Design review of the part built by this model. Coordinates are the model's own, in mm. Face numbers are marked on the shaded views. A direction names the side the tool comes from. Round coordinates to 2 decimals unless told otherwise and drop trailing zeros. Write each loop counter-clockwise with the first axis right and the second up, starting at its lowest first coordinate (ties: lowest second). Pieces come first, ordered by that corner, then holes. Notation, with made-up numbers: M 82.5,66 L 100.5,66 A29 ccw 100.5,98 Z; hole C -35.75,-25 d7. An arc over 180 degrees is marked long. One line per question, with ' | ' between items. Start each with the question number.
Item 1: Machinability: for the marked faces 4 and 5, which of the approach directions +Z, -Z, +X, -X, +Y, -Y give a long, thin tool a straight path to every point of the face, cutting with its end or side? Answer none if there is none.
Item 2: Add section D-D, the plane x = 27.5. State the section outline as (y, z) points, and give its area (3 significant figures).
Item 3: For L1, parallel to X at y = 6.25, z = -17; L2, parallel to Z at x = -14, y = 19.5; L3, parallel to Z at x = -19.5, y = 15.75, list the stretches that pass through material, from the lowest coordinate up.
Item 4: Add section A-A, the plane z = 0. State the section outline as (x, y) points, and give its area (3 significant figures).
Item 5: Draft analysis for pull direction Z (two halves, no side actions). For the marked faces 1, 2 and 3, state which applies: released by +Z, released by -Z, zero draft, split by the parting line, or undercut.
Item 6: Insertion check: pin 1 Ø2.5 at (y, z) = (9.5, -24.5) entering from +X; pin 2 Ø5 at (y, z) = (13, 24.5) entering from +X; pin 3 Ø1.4 at (y, z) = (18, 24) entering from -X. Each pin has a flat end and moves straight along its axis. Give the tip position at first contact, or say it passes through.
Item 7: Add section B-B, the plane y = 7.25. Give the number of separate pieces and of enclosed holes in the cut face, and give its area (3 significant figures).
Item 8: Add section C-C, the plane x = 4.5. State the section outline as (y, z) points, and give its area (3 significant figures).
```python
from build123d import *

# Parameters (mm, degrees)
SKETCH1_R           = 2.01295
BOSS_EXTRUDE1_DEPTH = 25.4


with BuildPart() as part:
    # Sketch1 → Boss-Extrude1 (new body)
    with BuildSketch(Plane(origin=(0, 0, 0), x_dir=(1, 0, 0), z_dir=(0, 1, 0))):
        with BuildLine():
            ThreePointArc((32.16275, -21.451406337), (28.205815008, -27.54883493), (22.589075945, -32.16275))
            Line((22.589075945, -32.16275), (-22.589075945, -32.16275))
            ThreePointArc((-22.589075945, -32.16275), (-28.205815008, -27.54883493), (-32.16275, -21.451406337))
            Line((-32.16275, -21.451406337), (-32.16275, 21.451406337))
            ThreePointArc((-32.16275, 21.451406337), (-28.205815008, 27.54883493), (-22.589075945, 32.16275))
            Line((-22.589075945, 32.16275), (22.589075945, 32.16275))
            ThreePointArc((22.589075945, 32.16275), (28.205815008, 27.54883493), (32.16275, 21.451406337))
            Line((32.16275, 21.451406337), (32.16275, -21.451406337))
        make_face()
        with Locations((-28.4734, 0)):
            Circle(SKETCH1_R, mode=Mode.SUBTRACT)
        with Locations((28.4734, 0)):
            Circle(SKETCH1_R, mode=Mode.SUBTRACT)
        with BuildLine():
            Line((3.466558561, -21.451406337), (3.466558561, -26.02865))
            Line((3.466558561, -26.02865), (26.02865, -26.02865))
            Line((26.02865, -26.02865), (26.02865, -4.794756681))
            ThreePointArc((26.02865, -4.794756681), (23.812095234, 0), (26.02865, 4.794756681))
            Line((26.02865, 4.794756681), (26.02865, 26.02865))
            Line((26.02865, 26.02865), (3.466558561, 26.02865))
            Line((3.466558561, 26.02865), (3.466558561, 21.451406337))
            ThreePointArc((3.466558561, 21.451406337), (14.879452296, 15.836090473), (21.194106975, 4.794756681))
            Line((21.194106975, 4.794756681), (18.856346659, 4.794756681))
            ThreePointArc((18.856346659, 4.794756681), (0, 19.4564), (-18.856346659, 4.794756681))
            Line((-18.856346659, 4.794756681), (-21.194106975, 4.794756681))
            ThreePointArc((-21.194106975, 4.794756681), (-14.879452296, 15.836090473), (-3.466558561, 21.451406337))
            Line((-3.466558561, 21.451406337), (-3.466558561, 26.02865))
            Line((-3.466558561, 26.02865), (-26.02865, 26.02865))
            Line((-26.02865, 26.02865), (-26.02865, 4.794756681))
            ThreePointArc((-26.02865, 4.794756681), (-23.812095234, 0), (-26.02865, -4.794756681))
            Line((-26.02865, -4.794756681), (-26.02865, -26.02865))
            Line((-26.02865, -26.02865), (-3.466558561, -26.02865))
            Line((-3.466558561, -26.02865), (-3.466558561, -21.451406337))
            ThreePointArc((-3.466558561, -21.451406337), (-14.879452296, -15.836090473), (-21.194106975, -4.794756681))
            Line((-21.194106975, -4.794756681), (-18.856346659, -4.794756681))
            ThreePointArc((-18.856346659, -4.794756681), (0, -19.4564), (18.856346659, -4.794756681))
            Line((18.856346659, -4.794756681), (21.194106975, -4.794756681))
            ThreePointArc((21.194106975, -4.794756681), (14.879452296, -15.836090473), (3.466558561, -21.451406337))
        make_face(mode=Mode.SUBTRACT)
    extrude(amount=BOSS_EXTRUDE1_DEPTH)


solid = part.part
```
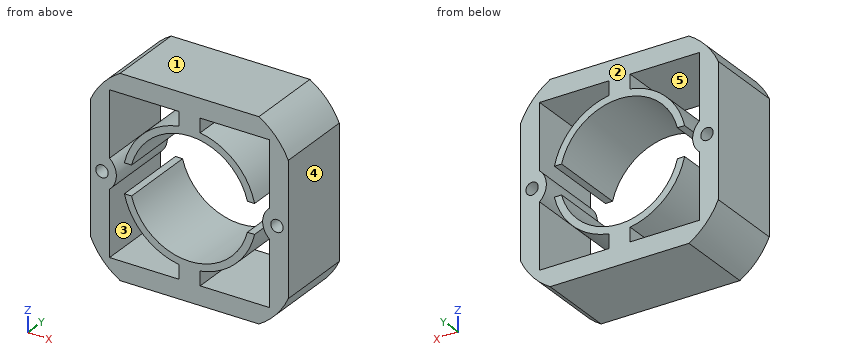
Computed values:
1) face 4: +Z, -Z, +X, +Y, -Y | face 5: +Y, -Y
2) outline: M 0,-28.3 L 25.4,-28.3 L 25.4,-1.76 L 0,-1.76 Z; M 0,1.76 L 25.4,1.76 L 25.4,28.3 L 0,28.3 Z | area: 1,350 mm^2
3) L1: x = -32.16 to -26.03, -13.53 to -9.46, 9.46 to 13.53, 26.03 to 32.16 | L2: z = -32.16 to -26.03, -16.62 to -13.51, 13.51 to 16.62, 26.03 to 32.16 | L3: z = -32.16 to -26.03, -9.59 to -4.79, 4.79 to 9.59, 26.03 to 32.16
4) outline: M -32.16,0 L -30.49,0 L -30.49,25.4 L -32.16,25.4 Z; M -26.46,0 L -23.81,0 L -23.81,25.4 L -26.46,25.4 Z; M 23.81,0 L 26.46,0 L 26.46,25.4 L 23.81,25.4 Z; M 30.49,0 L 32.16,0 L 32.16,25.4 L 30.49,25.4 Z | area: 220 mm^2
5) face 1: released by +Z | face 2: zero draft | face 3: undercut
6) pin 1: stops at x = 31.26 | pin 2: stops at x = 31.91 | pin 3: stops at x = -31.23
7) separate pieces: 1 | enclosed holes: 3 | area: 1,580 mm^2
8) outline: M 0,-32.16 L 25.4,-32.16 L 25.4,-26.03 L 0,-26.03 Z; M 0,-21.26 L 25.4,-21.26 L 25.4,-18.93 L 0,-18.93 Z; M 0,18.93 L 25.4,18.93 L 25.4,21.26 L 0,21.26 Z; M 0,26.03 L 25.4,26.03 L 25.4,32.16 L 0,32.16 Z | area: 430 mm^2
